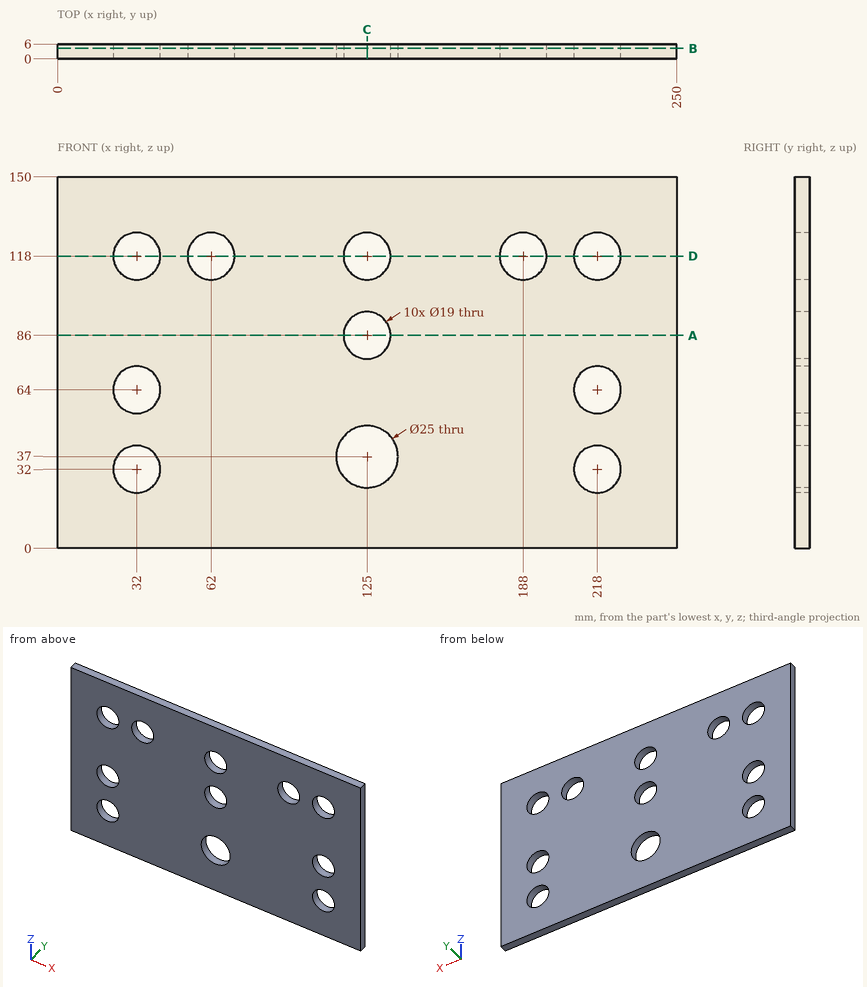
Drawing for the job (mm, zero at the part's lowest x, y, z). Round coordinates to 2 decimals unless told otherwise and drop trailing zeros. Write each loop counter-clockwise with the first axis right and the second up, starting at its lowest first coordinate (ties: lowest second). Pieces come first, ordered by that corner, then holes.
Item 1: Band-saw the part on C-C on x = 125. Write the cut outline in (y, z).
Filled in:
outline: (0, 0) - (6, 0) - (6, 24.5) - (0, 24.5) - close; (0, 49.5) - (6, 49.5) - (6, 76.5) - (0, 76.5) - close; (0, 95.5) - (6, 95.5) - (6, 108.5) - (0, 108.5) - close; (0, 127.5) - (6, 127.5) - (6, 150) - (0, 150) - close
Item 2: Band-saw the part on D-D on z = 118. Write the cut outline in (x, y), then the cut area to 3 significant figures.
Filled in:
outline: (0, 0) - (22.5, 0) - (22.5, 6) - (0, 6) - close; (41.5, 0) - (52.5, 0) - (52.5, 6) - (41.5, 6) - close; (71.5, 0) - (115.5, 0) - (115.5, 6) - (71.5, 6) - close; (134.5, 0) - (178.5, 0) - (178.5, 6) - (134.5, 6) - close; (197.5, 0) - (208.5, 0) - (208.5, 6) - (197.5, 6) - close; (227.5, 0) - (250, 0) - (250, 6) - (227.5, 6) - close
area: 930 mm2
Item 3: Drill centre lines: L1, parallel to Z at x = 218, y = 4; L2, parallel to Z at x = 125, y = 1.9; L3, parallel to X at y = 3.15, z = 70. Where is each one in solid material? Low to high.
Filled in:
L1: z = 0 to 22.5, 41.5 to 54.5, 73.5 to 108.5, 127.5 to 150
L2: z = 0 to 24.5, 49.5 to 76.5, 95.5 to 108.5, 127.5 to 150
L3: x = 0 to 24.63, 39.37 to 210.63, 225.37 to 250
Item 4: Band-saw the part on A-A on z = 86. Write the cut outline in (x, y), then the cut area to 3 significant figures.
Filled in:
outline: (0, 0) - (115.5, 0) - (115.5, 6) - (0, 6) - close; (134.5, 0) - (250, 0) - (250, 6) - (134.5, 6) - close
area: 1,390 mm2
Item 5: Band-saw the part on B-B on y = 4.2. Give the number of separate pieces and of enclosed holes in the cut face, then the cut area to 3 significant figures.
Filled in:
separate pieces: 1
enclosed holes: 11
area: 34,200 mm2
